For this review, take the finished solid that the model builds, in its own axes (mm). Face numbers are marked on the shaded views. A direction names the side the tool comes from. Coordinates: 2 decimals unless noted, no trailing zeros. Write each loop counter-clockwise with the first axis right and the second up, starting at its lowest first coordinate (ties: lowest second). Pieces come first, ordered by that corner, then holes.
```python
from build123d import *

# Parameters (mm, degrees)
SKETCH1_W           = 76.206980413
SKETCH1_H           = 76.206980413
BOSS_EXTRUDE1_DEPTH = 76.2
FILLET1_R           = 15.24
FILLET4_R           = 38.10349
CUT_EXTRUDE1_DEPTH  = 207.518
SKETCH4_R           = 12.615490026
BOSS_EXTRUDE2_DEPTH = 25.4


with BuildPart() as part:
    # Sketch1 → Boss-Extrude1 (new body)
    with BuildSketch(Plane.XY):
        with Locations((38.103490207, 38.103490207)):
            Rectangle(SKETCH1_W, SKETCH1_H)
    extrude(amount=BOSS_EXTRUDE1_DEPTH)

    # Fillet1
    fillet1_edges = [part.edges().sort_by_distance(p)[0] for p in [
        (38.103490206, 0, 76.2),
        (38.103490206, 0, 0),
    ]]
    fillet(fillet1_edges, radius=FILLET1_R)

    # Fillet4
    fillet4_edges = [part.edges().sort_by_distance(p)[0] for p in [
        (76.206980413, 76.206980413, 38.1),
        (0, 76.206980413, 38.1),
    ]]
    fillet(fillet4_edges, radius=FILLET4_R)

    # Sketch3 → Cut-Extrude1 (cut)
    with BuildSketch(Plane(origin=(76.206980413, 0, 0), x_dir=(0, 0, -1), z_dir=(1, 0, 0))):
        with BuildLine():
            Line((-71.12, 76.206980413), (-5.08, 76.206980413))
            Line((-5.08, 76.206980413), (-5.08, 38.103490206))
            Line((-5.08, 38.103490206), (-5.08, 15.24))
            ThreePointArc((-5.08, 15.24), (-8.055795103, 8.055795103), (-15.24, 5.08))
            Line((-15.24, 5.08), (-60.96, 5.08))
            ThreePointArc((-60.96, 5.08), (-68.144204897, 8.055795103), (-71.12, 15.24))
            Line((-71.12, 15.24), (-71.12, 38.103490206))
            Line((-71.12, 38.103490206), (-71.12, 76.206980413))
        make_face()
    extrude(amount=-CUT_EXTRUDE1_DEPTH, mode=Mode.SUBTRACT)

    # Sketch4 → Boss-Extrude2 (add)
    with BuildSketch(Plane(origin=(0, 0, 0), x_dir=(-1, 0, 0), z_dir=(0, -1, 0))):
        with Locations((-37.114040008, -37.351744978)):
            Circle(SKETCH4_R)
    extrude(amount=BOSS_EXTRUDE2_DEPTH)


solid = part.part
```
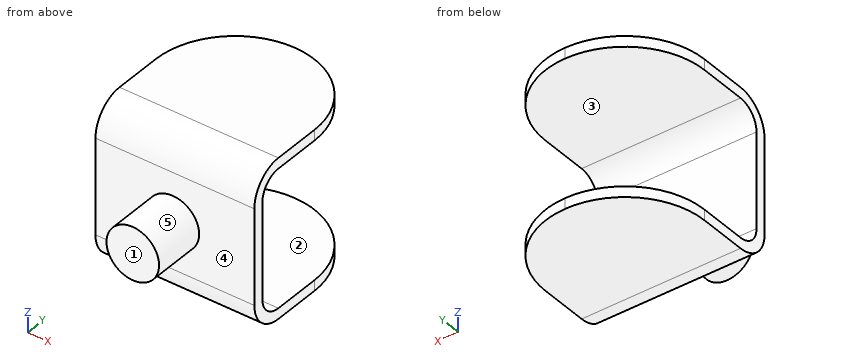
Q1. Add section C-C (x = 56.5). State the section outline as (y, z) points.
Ans:
outline: (0, 15.24) arc R15.24 ccw to (15.24, 0) - (71.47, 0) - (71.47, 5.08) - (15.24, 5.08) arc R10.16 cw to (5.08, 15.24) - (5.08, 60.96) arc R10.16 cw to (15.24, 71.12) - (71.47, 71.12) - (71.47, 76.2) - (15.24, 76.2) arc R15.24 ccw to (0, 60.96) - close
Q2. For probe 1 along Z at (x, y) = (45, 15); probe 2 along Y at (x, z) = (57, 35); probe 3 along X at (y, z) = (-8, 38), list the stretches that pass through material, from the lowest coordinate up.
Ans:
probe 1: z = 0 to 5.08, 71.12 to 76.2
probe 2: y = 0 to 5.08
probe 3: x = 24.52 to 49.71
Q3. Add section D-D (y = 8.5). State the section outline as (x, z) points.
Ans:
outline: (0, 1.57) - (76.21, 1.57) - (76.21, 7.64) - (0, 7.64) - close; (0, 68.56) - (76.21, 68.56) - (76.21, 74.63) - (0, 74.63) - close
Q4. Tool access review of the marked faces 1 and 2: name each direction out of +Z, -Z, +X, -X, +Y, -Y from which nothing blocks a thin tool from reaching the whole face with its end or side.
Ans:
face 1: +Z, -Z, +X, -X, -Y
face 2: +X, -X, +Y
Q5. Add section B-B (z = 44.5). State the section outline as (x, y) points.
Ans:
outline: (0, 0) - (26.72, 0) - (26.72, -25.4) - (47.51, -25.4) - (47.51, 0) - (76.21, 0) - (76.21, 5.08) - (0, 5.08) - close
Q6. Draft analysis for pull direction Z (two halves, no side actions). For the marked faces 3, 4 and 5, state which applies: +Z half, -Z half, draft (parallel to the pull), parting line (faces both ways), or undercut.
Ans:
face 3: undercut
face 4: draft
face 5: parting line
Q7. Clearance check with flat-ended pins moving along their axes: pin 1 Ø6 at (x, z) = (50, 48) entering from -Y; pin 2 Ø3 at (x, y) = (36, -12) entering from -Z; pin 3 Ø5 at (x, y) = (55, 9.5) entering from -Z; pin 4 Ø5 at (y, z) = (-1.5, 25) entering from -X. State where each tip first meets the part, or that it passes through.
Ans:
pin 1: stops at y = 0
pin 2: stops at z = 24.74
pin 3: stops at z = 0.35
pin 4: stops at x = 0
Q8. Add section A-A (y = 20). State the section outline as (x, z) points, then the cut area to 3 significant figures.
Ans:
outline: (0, 0) - (76.21, 0) - (76.21, 5.08) - (0, 5.08) - close; (0, 71.12) - (76.21, 71.12) - (76.21, 76.2) - (0, 76.2) - close
area: 774 mm2
